from build123d import *

# Parameters (mm, degrees)
SKETCH1_R           = 1.5
BOSS_EXTRUDE1_DEPTH = 150


with BuildPart() as part:
    # Sketch1 → Boss-Extrude1 (new body)
    with BuildSketch(Plane(origin=(0, 0, 0), x_dir=(1, 0, 0), z_dir=(0, 1, 0))):
        with Locations(Location((0, 0, 0), (0, 0, 270))):
            Circle(SKETCH1_R)
    extrude(amount=BOSS_EXTRUDE1_DEPTH)

    # Sketch2 → Revolve1 (revolve)
    with BuildSketch(Plane(origin=(0, 0, 0), x_dir=(0, 0, -1), z_dir=(1, 0, 0))):
        with BuildLine():
            Line((0, 5), (0, -5))
            ThreePointArc((0, -5), (5, 0), (0, 5))
        make_face()
    revolve1 = revolve(axis=Axis((0, 5, 0), (0, -1, 0)))

    # Mirror1: Revolve1 across plane
    add(revolve1.mirror(Plane.ZX.offset(75)))


solid = part.part
Input: part model. Units: mm. Frame: model coordinates. Round coordinates to 2 decimals unless told otherwise and drop trailing zeros. Loops run counter-clockwise (first coordinate to the right, second up) from the corner with the lowest first, then second, coordinate; pieces in that order, holes last. Notation, with made-up numbers: (13.5, 39) -> (61.5, 39) arc R30 cw to (61.5, 65) -> close; hole circle Ø11 at (78.25, 80.25). An arc over 180 degrees is marked (long way). Answer as a JSON object with one key per item and string values. Group by question number.
1) Ray query, L1, parallel to Y at x = -3.75, z = -2.5; L2, parallel to Y at x = -1, z = -4.5; L3, parallel to Z at x = 0, y = 140.5. Return the intervals inside material, ascending.
2) Pin query (flat end, axial travel): pin 1 (4 mm diameter, centred on y = 30.5, z = 4, fed in from -X); pin 2 (3 mm diameter, centred on x = 1.5, z = -3, fed in from -Y); pin 3 (4 mm diameter, centred on y = 69.5, z = -2.5, fed in from -X). Return the tip coordinate at first contact, or that it passes through.
3) Section query A-A on x = 0. Output: boundary loops of the cut face in (y, z), plus the area to 3 significant figures.
4) Section query B-B on z = -3.5. Output: boundary loops of the cut face in (x, y), plus the area to 3 significant figures.
5) Section query C-C on y = 23. Output: boundary loops of the cut face in (x, z), plus the area to 3 significant figures.
Reply:
{
 "1": {"L1": "y = -2.17 to 2.17, 147.83 to 152.17", "L2": "y = -1.94 to 1.94, 148.06 to 151.94", "L3": "z = -1.5 to 1.5"},
 "2": {"pin 1": "passes through", "pin 2": "stops at y = -4.64", "pin 3": "stops at x = -1.41"},
 "3": {"outline": "(4.77, -1.5) -> (145.23, -1.5) arc R5 ccw (long way) to (145.23, 1.5) -> (4.77, 1.5) arc R5 ccw (long way) to start", "area": "578 mm2"},
 "4": {"outline": "circle Ø7.14 at (0, 0); circle Ø7.14 at (0, 150)", "area": "80.1 mm2"},
 "5": {"outline": "circle Ø3 at (0, 0)", "area": "7.07 mm2"}
}
